Could you check a few things on this drawing? It's one solid part, dimensions in mm from its lowest x, y, z. A direction names the side the tool comes from. Give positions to 0.01 mm unless a question says otherwise; leave off trailing zeros. Write each loop counter-clockwise with the first axis right and the second up, starting at its lowest first coordinate (ties: lowest second). Pieces come first, ordered by that corner, then holes.
1. Suppose I cut it at D-D (x = 50.8). Please give me the cut outline in (y, z), and give its area (3 significant figures).
2. On a 3-axis mill with a long thin cutter (end or side, diameter ignored), from which of +Z, -Z, +X, -X, +Y, -Y can I reach the whole of each face in a straight line? I mean the marked faces 4, 5 and 6. Say none if no direction works.
3. If I drill on probe 1 along Y at (x, z) = (5, 38); probe 2 along X at (y, z) = (25, 61.5); probe 3 along Z at (x, y) = (94, 25), over which ranges is the centre line in solid material (lowest first)?
4. Suppose I cut it at A-A (y = 25.4). Please give me the cut outline in (x, z).
5. Suppose I cut it at C-C (x = 8). Please give me the cut outline in (y, z).
6. Thinking about a two-plate mould opening in Z: for the marked faces 1, 2 and 3, which applies, pulls with the +Z half, pulls with the -Z half, needs draft (parallel to the pull), parting line crosses it, or undercut?
7. I'm going to push flat-ended pins straight in: pin 1 (23 mm diameter, centred on x = 42.5, z = 42.5, fed in from -Y); pin 2 (6 mm diameter, centred on y = 125.5, z = 38.5, fed in from +X); pin 3 (8 mm diameter, centred on x = 31, z = 63.5, fed in from +Y). Where does each tip first touch, or does it pass through?
8. Suppose I cut it at B-B (z = 38.1). Please give me the cut outline in (x, y).
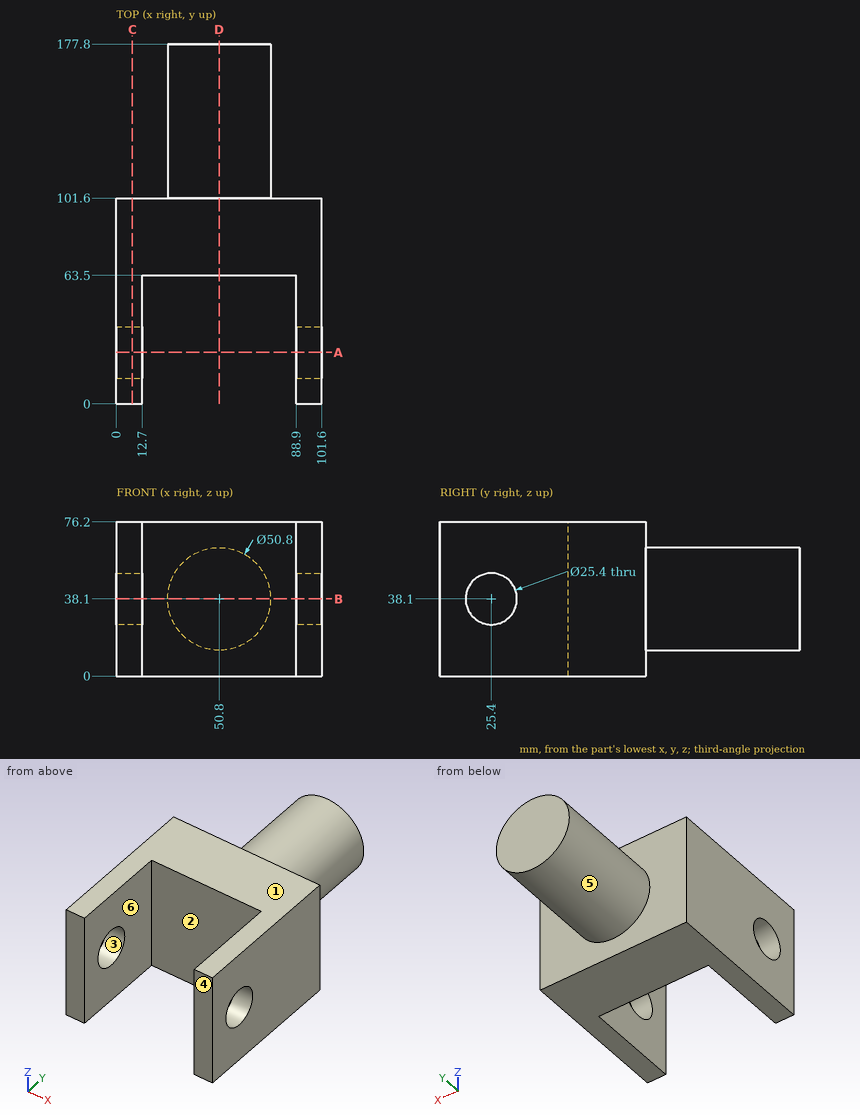
Checks:
1. outline: (63.5, 0) - (101.6, 0) - (101.6, 12.7) - (177.8, 12.7) - (177.8, 63.5) - (101.6, 63.5) - (101.6, 76.2) - (63.5, 76.2) - close
1. area: 6,770 mm2
2. face 4: +Z, -Z, +X, -X, -Y
2. face 5: +Y
2. face 6: +Z, -Z, -Y
3. probe 1: y = 0 to 12.7, 38.1 to 101.6
3. probe 2: x = 0 to 12.7, 88.9 to 101.6
3. probe 3: z = 0 to 25.41, 50.79 to 76.2
4. outline: (0, 0) - (12.7, 0) - (12.7, 25.4) - (0, 25.4) - close; (0, 50.8) - (12.7, 50.8) - (12.7, 76.2) - (0, 76.2) - close; (88.9, 0) - (101.6, 0) - (101.6, 25.4) - (88.9, 25.4) - close; (88.9, 50.8) - (101.6, 50.8) - (101.6, 76.2) - (88.9, 76.2) - close
5. outline: (0, 0) - (101.6, 0) - (101.6, 76.2) - (0, 76.2) - close; hole circle Ø25.4 at (25.4, 38.1)
6. face 1: pulls with the +Z half
6. face 2: needs draft
6. face 3: undercut
7. pin 1: stops at y = 63.5
7. pin 2: stops at x = 76.2
7. pin 3: stops at y = 101.6
8. outline: (0, 0) - (12.7, 0) - (12.7, 12.7) - (0, 12.7) - close; (0, 38.1) - (12.7, 38.1) - (12.7, 63.5) - (88.9, 63.5) - (88.9, 38.1) - (101.6, 38.1) - (101.6, 101.6) - (76.2, 101.6) - (76.2, 177.8) - (25.4, 177.8) - (25.4, 101.6) - (0, 101.6) - close; (88.9, 0) - (101.6, 0) - (101.6, 12.7) - (88.9, 12.7) - close
